Part model, mm, in its own coordinate system. A direction names the side the tool comes from. Round coordinates to 2 decimals unless told otherwise and drop trailing zeros. Loops run counter-clockwise (first coordinate to the right, second up) from the corner with the lowest first, then second, coordinate; pieces in that order, holes last.
(1) Mould opens along Z. For faces 6 (the face through (-42, 15, -15)), 7 (the face through (43.2, 15, -16)), 8 (the face through (44, 15, 59)) say: +Z half, -Z half, draft (parallel to the pull), parting line (faces both ways), or undercut.
(2) Cut at C-C on y = 21. List the corners of the cut face in (x, z), then the cut area to 3 significant figures.
(3) Probe probe 1 along Z at (x, y) = (46.5, 21.5); probe 2 along Z at (x, y) = (-15, 1.55); probe 3 along Z at (x, y) = (15, 2.05). List the from-to ranges inside material, lowest first.
(4) Cut at D-D on z = 35.5. List the corners of the cut face in (x, y), then the cut area to 3 significant figures.
(5) Cut at A-A on y = 10.75. List the corners of the cut face in (x, z).
(6) Tool access for faces 1 (the face through (45, 15, 51)), 2 (the face through (-45, 15, -85)), 3 (the face through (-15.8, 1.5, 90.5)), 4 (the face through (-34, 6, 24)), 5 (the face through (0, 3, 24)): list every direction of +Z, -Z, +X, -X, +Y, -Y with a clear straight run to the whole face (end or side of a thin tool).
(7) Cut at B-B on x = -2.5. List the corners of the cut face in (y, z).
(8) Flat gauge pins, fed straight in: pin 1 (3.5 mm diameter, centred on y = 5, z = -63, fed in from +X); pin 2 (2 mm diameter, centred on x = 38.5, y = 11.5, fed in from +Z); pin 3 (10 mm diameter, centred on x = 25, z = 20, fed in from +Y); pin 4 (2.5 mm diameter, centred on y = 4, z = 25.5, fed in from -X). Where does each tip first touch, or does it go through?
from build123d import *

# Parameters (mm, degrees)
SCHIZZO1_W                    = 101
SCHIZZO1_H                    = 186
ESTRUSIONE_ESTRUSIONE1_DEPTH  = 3
ESTRUSIONE_ESTRUSIONE3_DEPTH  = 25
SCHIZZO2_W                    = 70
SCHIZZO2_H                    = 50
SCHIZZO2_W_2                  = 67.6
SCHIZZO2_H_2                  = 47.6
ESTRUSIONE_ESTRUSIONE2_DEPTH  = 3
ESTRUSIONE_ESTRUSIONE5_DEPTH  = 70
TAGLIO_ESTRUSIONE2_DEPTH      = 109.739367296
TAGLIO_ESTRUSIONE2_DEPTH_BACK = 109.739367296
SCHIZZO9_R                    = 7.5
SCHIZZO4_W                    = 7.2
SCHIZZO4_H                    = 1.8
TAGLIO_ESTRUSIONE1_DEPTH      = 109.739367296
ESTRUSIONE_ESTRUSIONE4_DEPTH  = 25
FORO_2_8_2_8_1_D              = 2.8
FORO_2_8_2_8_1_DEPTH          = 10
FORO_2_8_2_8_1_TIP            = 0.841204867
SMUSSO1_SIZE                  = 20
SMUSSO1_SIZE2                 = 34.641016151
RACCORDO1_R                   = 4
TAGLIO_ESTRUSIONE3_DEPTH      = 109.739367296
FORO_PER_VITE_M3_1_D          = 3.4
FORO_PER_VITE_M3_1_DEPTH      = 10
FORO_PER_VITE_M3_1_TIP        = 1.021463052


with BuildPart() as part:
    # Schizzo1 → Estrusione-Estrusione1 (new body)
    with BuildSketch(Plane(origin=(0, 0, 0), x_dir=(1, 0, 0), z_dir=(0, 1, 0))):
        Rectangle(SCHIZZO1_W, SCHIZZO1_H)
    extrude(amount=ESTRUSIONE_ESTRUSIONE1_DEPTH)

    # Schizzo3 → Estrusione-Estrusione3 (add)
    with BuildSketch(Plane(origin=(0, 3, 0), x_dir=(1, 0, 0), z_dir=(0, 1, 0))):
        Polygon((-43.2, -59), (-42, -59), (-42, 91.8), (42, 91.8), (42, -59), (43.2, -59), (43.2, 93), (-43.2, 93), align=None)
    extrude(amount=ESTRUSIONE_ESTRUSIONE3_DEPTH)

    # Schizzo2 → Estrusione-Estrusione2 (add)
    # profile 1 of 2: a face of its own
    with BuildSketch(Plane(origin=(0, 3, 0), x_dir=(1, 0, 0), z_dir=(0, 1, 0))):
        with Locations((0, 51)):
            Rectangle(SCHIZZO2_W, SCHIZZO2_H)
        with Locations((0, 51)):
            Rectangle(SCHIZZO2_W_2, SCHIZZO2_H_2, mode=Mode.SUBTRACT)
    # profile 2 of 2: a face of its own
    with BuildSketch(Plane(origin=(0, 3, 0), x_dir=(1, 0, 0), z_dir=(0, 1, 0))):
        with Locations((0, -24)):
            Rectangle(SCHIZZO2_W, SCHIZZO2_H)
        with Locations((0, -24)):
            Rectangle(SCHIZZO2_W_2, SCHIZZO2_H_2, mode=Mode.SUBTRACT)
    extrude(amount=ESTRUSIONE_ESTRUSIONE2_DEPTH)

    # Schizzo13 → Estrusione-Estrusione5 (add)
    with BuildSketch(Plane.ZY.offset(35)):
        Polygon((49, 6), (57.5, 3), (49, 3), align=None)
    extrude(amount=-ESTRUSIONE_ESTRUSIONE5_DEPTH)

    # Schizzo9 → Taglio-Estrusione2 (cut, two sides: drawn at the far end of the back side and taken through both)
    with BuildSketch(Plane(origin=(0, 3, 0), x_dir=(1, 0, 0), z_dir=(0, 1, 0)).offset(-TAGLIO_ESTRUSIONE2_DEPTH_BACK)):
        with Locations(Location((0, -36.2, 0), (0, 0, 270))):
            Circle(SCHIZZO9_R)
    extrude(amount=TAGLIO_ESTRUSIONE2_DEPTH + TAGLIO_ESTRUSIONE2_DEPTH_BACK, mode=Mode.SUBTRACT)

    # Schizzo4 → Taglio-Estrusione1 (cut, through all)
    with BuildSketch(Plane(origin=(0, 3, 0), x_dir=(1, 0, 0), z_dir=(0, 1, 0))):
        with Locations((13, -58.9)):
            Rectangle(SCHIZZO4_W, SCHIZZO4_H)
    extrude(amount=-TAGLIO_ESTRUSIONE1_DEPTH, mode=Mode.SUBTRACT)

    # Schizzo5 → Estrusione-Estrusione4 (add)
    with BuildSketch(Plane(origin=(0, 3, 0), x_dir=(1, 0, 0), z_dir=(0, 1, 0))):
        with BuildLine():
            Line((-43.2, 93), (-43.2, 85))
            Line((-43.2, 85), (-46.5, 85))
            ThreePointArc((-46.5, 85), (-50.5, 89), (-46.5, 93))
            Line((-46.5, 93), (-43.2, 93))
        make_face()
        with BuildLine():
            Line((46.5, 85), (43.2, 85))
            Line((43.2, 85), (43.2, 93))
            Line((43.2, 93), (46.5, 93))
            ThreePointArc((46.5, 93), (50.5, 89), (46.5, 85))
        make_face()
        with BuildLine():
            Line((46.5, -51), (43.2, -51))
            Line((43.2, -51), (43.2, -59))
            Line((43.2, -59), (46.5, -59))
            ThreePointArc((46.5, -59), (50.5, -55), (46.5, -51))
        make_face()
        with BuildLine():
            Line((-46.5, -51), (-43.2, -51))
            Line((-43.2, -51), (-43.2, -59))
            Line((-43.2, -59), (-46.5, -59))
            ThreePointArc((-46.5, -59), (-50.5, -55), (-46.5, -51))
        make_face()
    extrude(amount=ESTRUSIONE_ESTRUSIONE4_DEPTH)

    # Foro Ø2.8 (2.8)-1
    with Locations(Plane(origin=(0, 28, 0), x_dir=(1, 0, 0), z_dir=(0, 1, 0))):
        with Locations((-46.5, 89), (46.5, 89), (46.5, -55), (-46.5, -55)):
            Hole(FORO_2_8_2_8_1_D / 2, depth=FORO_2_8_2_8_1_DEPTH)
            with Locations((0, 0, -(FORO_2_8_2_8_1_DEPTH + FORO_2_8_2_8_1_TIP / 2))):  # 118° drill point
                Cone(0, FORO_2_8_2_8_1_D / 2, FORO_2_8_2_8_1_TIP, mode=Mode.SUBTRACT)

    # Smusso1
    smusso1_edges = [part.edges().sort_by_distance(p)[0] for p in [
        (50.5, 1.5, 93),
        (-50.5, 1.5, 93),
    ]]
    smusso1_side = [part.faces().sort_by_distance(p)[0] for p in [
        (0, 1.5, 93),
    ]]
    chamfer(smusso1_edges, length=SMUSSO1_SIZE, length2=SMUSSO1_SIZE2, reference=smusso1_side[0])

    # Raccordo1
    raccordo1_edges = [part.edges().sort_by_distance(p)[0] for p in [
        (50.5, 1.5, 58.358983849),
        (-50.5, 1.5, 58.358983849),
        (30.5, 1.5, 93),
        (-30.5, 1.5, 93),
        (-50.5, 1.5, -93),
        (50.5, 1.5, -93),
    ]]
    fillet(raccordo1_edges, radius=RACCORDO1_R - 0.0001)  # a hair under: the kernel refuses the full size

    # Schizzo10 → Taglio-Estrusione3 (cut, through all)
    with BuildSketch(Plane(origin=(0, 3, 0), x_dir=(1, 0, 0), z_dir=(0, 1, 0))):
        with BuildLine():
            Line((29.25, 42.5), (29.25, 32.5))
            ThreePointArc((29.25, 32.5), (27.5, 30.75), (25.75, 32.5))
            Line((25.75, 32.5), (25.75, 42.5))
            ThreePointArc((25.75, 42.5), (27.5, 44.25), (29.25, 42.5))
        make_face()
        with BuildLine():
            Line((-25.75, 42.5), (-25.75, 32.5))
            ThreePointArc((-25.75, 32.5), (-27.5, 30.75), (-29.25, 32.5))
            Line((-29.25, 32.5), (-29.25, 42.5))
            ThreePointArc((-29.25, 42.5), (-27.5, 44.25), (-25.75, 42.5))
        make_face()
    extrude(amount=-TAGLIO_ESTRUSIONE3_DEPTH, mode=Mode.SUBTRACT)

    # Foro per Vite M3-1
    with Locations(Plane(origin=(0, 3, 0), x_dir=(1, 0, 0), z_dir=(0, 1, 0))):
        with Locations((15, -65), (15, -89), (-15, -89), (-15, -65)):
            Hole(FORO_PER_VITE_M3_1_D / 2, depth=FORO_PER_VITE_M3_1_DEPTH)
            with Locations((0, 0, -(FORO_PER_VITE_M3_1_DEPTH + FORO_PER_VITE_M3_1_TIP / 2))):  # 118° drill point
                Cone(0, FORO_PER_VITE_M3_1_D / 2, FORO_PER_VITE_M3_1_TIP, mode=Mode.SUBTRACT)


solid = part.part
Final values:
1. face 6: draft
1. face 7: undercut
1. face 8: +Z half
2. outline: (-46.5, -93) - (46.5, -93) arc R4 ccw to (46.5, -85) - (43.2, -85) - (43.2, 51) - (46.5, 51) arc R4 ccw to (46.5, 59) - (42, 59) - (42, -91.8) - (-42, -91.8) - (-42, 59) - (-46.5, 59) arc R4 ccw to (-46.5, 51) - (-43.2, 51) - (-43.2, -85) - (-46.5, -85) arc R4 ccw to start; hole circle Ø2.8 at (-46.5, -89); hole circle Ø2.8 at (-46.5, 55); hole circle Ø2.8 at (46.5, -89); hole circle Ø2.8 at (46.5, 55)
2. area: 647 mm2
3. probe 1: z = -93 to -90.4, -87.6 to -85, 51 to 53.6, 56.4 to 59
3. probe 2: z = -93 to 63.3, 66.7 to 87.3, 90.7 to 93
3. probe 3: z = -93 to 58, 59.8 to 63.3, 66.7 to 87.3, 90.7 to 93
4. outline: (-50.5, 0) - (-7.47, 0) - (-7.47, 3) - (-33.8, 3) - (-33.8, 6) - (-35, 6) - (-35, 3) - (-42, 3) - (-42, 28) - (-43.2, 28) - (-43.2, 3) - (-50.5, 3) - close; (7.47, 0) - (50.5, 0) - (50.5, 3) - (43.2, 3) - (43.2, 28) - (42, 28) - (42, 3) - (35, 3) - (35, 6) - (33.8, 6) - (33.8, 3) - (7.47, 3) - close
4. area: 325 mm2
5. outline: (-46.5, -93) - (46.5, -93) arc R4 ccw to (46.5, -85) - (43.2, -85) - (43.2, 51) - (46.5, 51) arc R4 ccw to (46.5, 59) - (42, 59) - (42, -91.8) - (-42, -91.8) - (-42, 59) - (-46.5, 59) arc R4 ccw to (-46.5, 51) - (-43.2, 51) - (-43.2, -85) - (-46.5, -85) arc R4 ccw to start
6. face 1: +X, +Y
6. face 2: -X, +Y
6. face 3: +Y, -Y
6. face 4: +Z, +Y
6. face 5: +Y
7. outline: (0, -93) - (28, -93) - (28, -91.8) - (3, -91.8) - (3, -76) - (6, -76) - (6, -74.8) - (3, -74.8) - (3, -27.2) - (6, -27.2) - (6, -26) - (3, -26) - (3, -1) - (6, -1) - (6, 0.2) - (3, 0.2) - (3, 29.13) - (0, 29.13) - close; (0, 43.27) - (3, 43.27) - (3, 47.8) - (6, 47.8) - (6, 49) - (3, 57.5) - (3, 93) - (0, 93) - close
8. pin 1: stops at x = 43.2
8. pin 2: stops at z = -91.8
8. pin 3: stops at y = 3
8. pin 4: stops at x = -50.5
